Check sheet for the modelled part. Datum: model origin and axes. Units: mm. Round coordinates to 2 decimals unless told otherwise and drop trailing zeros. Write each loop counter-clockwise with the first axis right and the second up, starting at its lowest first coordinate (ties: lowest second). Pieces come first, ordered by that corner, then holes.
Item 1: Cross-section at D-D on y = 28.5. Enter the section's corners in (x, z).
Item 2: Go/stop test with flat-tipped pins: pin 1 Ø2.5 at (y, z) = (9, 3) entering from -X; pin 2 Ø1.4 at (x, y) = (-74.5, 38.5) entering from -Z. Record where each tip stops, or that it passes through.
Item 3: Cross-section at B-B on y = 8.5. Enter the section's corners in (x, z), plus the area to 3 significant figures.
Item 4: Material ranges on line 1 (Y direction, x = -18.5, z = 0.2); line 2 (Y direction, x = -45, z = 2.55); line 3 (Y direction, x = 6, z = 1.9), recorded low to high.
Item 5: Cross-section at A-A on x = -51. Enter the section's corners in (y, z).
Item 6: Cross-section at C-C on x = -22.5. Enter the section's corners in (y, z).
from build123d import *

# Parameters (mm, degrees)
ESQUISSE1_R        = 1.5
ESQUISSE1_R_2      = 4.25
ESQUISSE1_R_3      = 1.2
ESQUISSE1_W        = 5
ESQUISSE1_H        = 5
BOSS_EXTRU_1_DEPTH = 5
CONG_1_R           = 5
CONG_2_R           = 10


with BuildPart() as part:
    # Esquisse1 → Boss.-Extru.1 (new body)
    with BuildSketch(Plane.XY):
        Polygon((-20, 0), (20, 0), (20, 6), (15, 6), (15, 11), (20, 11), (45.5, 11), (45.5, 46), (20, 46), (15, 46), (15, 51), (20, 51), (20, 57), (-20, 57), (-25, 57), (-65, 57), (-65, 51), (-60, 51), (-60, 46), (-65, 46), (-90.5, 46), (-90.5, 11), (-65, 11), (-60, 11), (-60, 6), (-65, 6), (-65, 0), (-25, 0), align=None)
        with Locations((0, 48.5)):
            Circle(ESQUISSE1_R, mode=Mode.SUBTRACT)
        with Locations((0, 8.5)):
            Circle(ESQUISSE1_R, mode=Mode.SUBTRACT)
        with Locations((0, 28.5)):
            Circle(ESQUISSE1_R_2, mode=Mode.SUBTRACT)
        with Locations(Location((-45, 8.5, 0), (0, 0, 180))):
            Circle(ESQUISSE1_R, mode=Mode.SUBTRACT)
        with Locations(Location((-45, 28.5, 0), (0, 0, 180))):
            Circle(ESQUISSE1_R_2, mode=Mode.SUBTRACT)
        with Locations(Location((-45, 48.5, 0), (0, 0, 180))):
            Circle(ESQUISSE1_R, mode=Mode.SUBTRACT)
        with Locations((6, 38.5)):
            Circle(ESQUISSE1_R_3, mode=Mode.SUBTRACT)
        with Locations(Location((6, 18.5, 0), (0, 0, 180))):
            Circle(ESQUISSE1_R_3, mode=Mode.SUBTRACT)
        with Locations((-51, 18.5)):
            Circle(ESQUISSE1_R_3, mode=Mode.SUBTRACT)
        with Locations(Location((-51, 38.5, 0), (0, 0, 180))):
            Circle(ESQUISSE1_R_3, mode=Mode.SUBTRACT)
        with Locations((35.5, 28.5)):
            Circle(ESQUISSE1_R_2, mode=Mode.SUBTRACT)
        with Locations(Location((-80.5, 28.5, 0), (0, 0, 180))):
            Circle(ESQUISSE1_R_2, mode=Mode.SUBTRACT)
        with Locations((29.5, 38.5)):
            Circle(ESQUISSE1_R_3, mode=Mode.SUBTRACT)
        with Locations(Location((29.5, 18.5, 0), (0, 0, 180))):
            Circle(ESQUISSE1_R_3, mode=Mode.SUBTRACT)
        with Locations((-74.5, 18.5)):
            Circle(ESQUISSE1_R_3, mode=Mode.SUBTRACT)
        with Locations(Location((-74.5, 38.5, 0), (0, 0, 180))):
            Circle(ESQUISSE1_R_3, mode=Mode.SUBTRACT)
        with Locations((-22.5, 28.5)):
            Circle(ESQUISSE1_R, mode=Mode.SUBTRACT)
        Polygon((-20, 51), (-15, 51), (-15, 46), (-20, 46), (-25, 46), (-30, 46), (-30, 51), (-25, 51), align=None, mode=Mode.SUBTRACT)
        Polygon((-20, 11), (-15, 11), (-15, 6), (-20, 6), (-25, 6), (-30, 6), (-30, 11), (-25, 11), align=None, mode=Mode.SUBTRACT)
        with Locations((-22.5, 21)):
            Rectangle(ESQUISSE1_W, ESQUISSE1_H, mode=Mode.SUBTRACT)
        with Locations((-22.5, 36)):
            Rectangle(ESQUISSE1_W, ESQUISSE1_H, mode=Mode.SUBTRACT)
    extrude(amount=BOSS_EXTRU_1_DEPTH)

    # Congé1
    cong_1_edges = [part.edges().sort_by_distance(p)[0] for p in [
        (-65, 0, 2.5),
        (-65, 57, 2.5),
        (20, 57, 2.5),
        (20, 0, 2.5),
    ]]
    fillet(cong_1_edges, radius=CONG_1_R)

    # Congé2
    cong_2_edges = [part.edges().sort_by_distance(p)[0] for p in [
        (-90.5, 11, 2.5),
        (-90.5, 46, 2.5),
        (45.5, 46, 2.5),
        (45.5, 11, 2.5),
    ]]
    fillet(cong_2_edges, radius=CONG_2_R)


solid = part.part
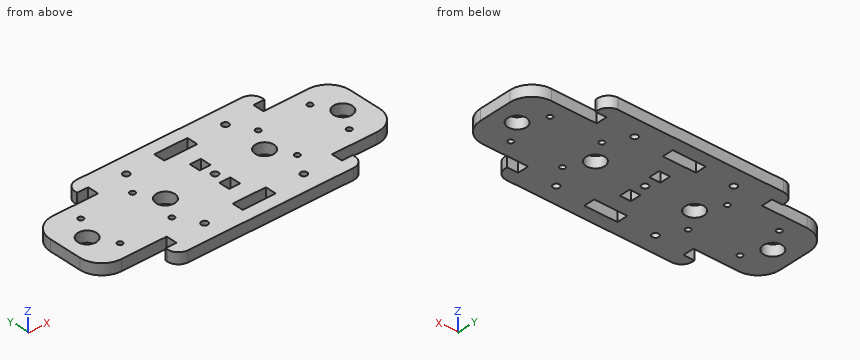
Response values:
1. outline: (-90.5, 0) - (-84.75, 0) - (-84.75, 5) - (-90.5, 5) - close; (-76.25, 0) - (-49.25, 0) - (-49.25, 5) - (-76.25, 5) - close; (-40.75, 0) - (-24, 0) - (-24, 5) - (-40.75, 5) - close; (-21, 0) - (-4.25, 0) - (-4.25, 5) - (-21, 5) - close; (4.25, 0) - (31.25, 0) - (31.25, 5) - (4.25, 5) - close; (39.75, 0) - (45.5, 0) - (45.5, 5) - (39.75, 5) - close
2. pin 1: stops at x = -60
2. pin 2: passes through
3. outline: (-60, 0) - (-46.5, 0) - (-46.5, 5) - (-60, 5) - close; (-43.5, 0) - (-30, 0) - (-30, 5) - (-43.5, 5) - close; (-15, 0) - (-1.5, 0) - (-1.5, 5) - (-15, 5) - close; (1.5, 0) - (15, 0) - (15, 5) - (1.5, 5) - close
3. area: 270 mm2
4. line 1: y = 0 to 6, 11 to 46, 51 to 57
4. line 2: y = 0 to 7, 10 to 24.25, 32.75 to 47, 50 to 57
4. line 3: y = 0 to 17.3, 19.7 to 37.3, 39.7 to 57
5. outline: (0, 0) - (17.3, 0) - (17.3, 5) - (0, 5) - close; (19.7, 0) - (37.3, 0) - (37.3, 5) - (19.7, 5) - close; (39.7, 0) - (57, 0) - (57, 5) - (39.7, 5) - close
6. outline: (0, 0) - (6, 0) - (6, 5) - (0, 5) - close; (11, 0) - (18.5, 0) - (18.5, 5) - (11, 5) - close; (23.5, 0) - (27, 0) - (27, 5) - (23.5, 5) - close; (30, 0) - (33.5, 0) - (33.5, 5) - (30, 5) - close; (38.5, 0) - (46, 0) - (46, 5) - (38.5, 5) - close; (51, 0) - (57, 0) - (57, 5) - (51, 5) - close
